Check sheet for the drawn part. Datum: minimum x, y, z corner. Units: mm. A direction names the side the tool comes from. Coordinates: 2 decimals unless noted, no trailing zeros. Loops run counter-clockwise (first coordinate to the right, second up) from the corner with the lowest first, then second, coordinate; pieces in that order, holes last.
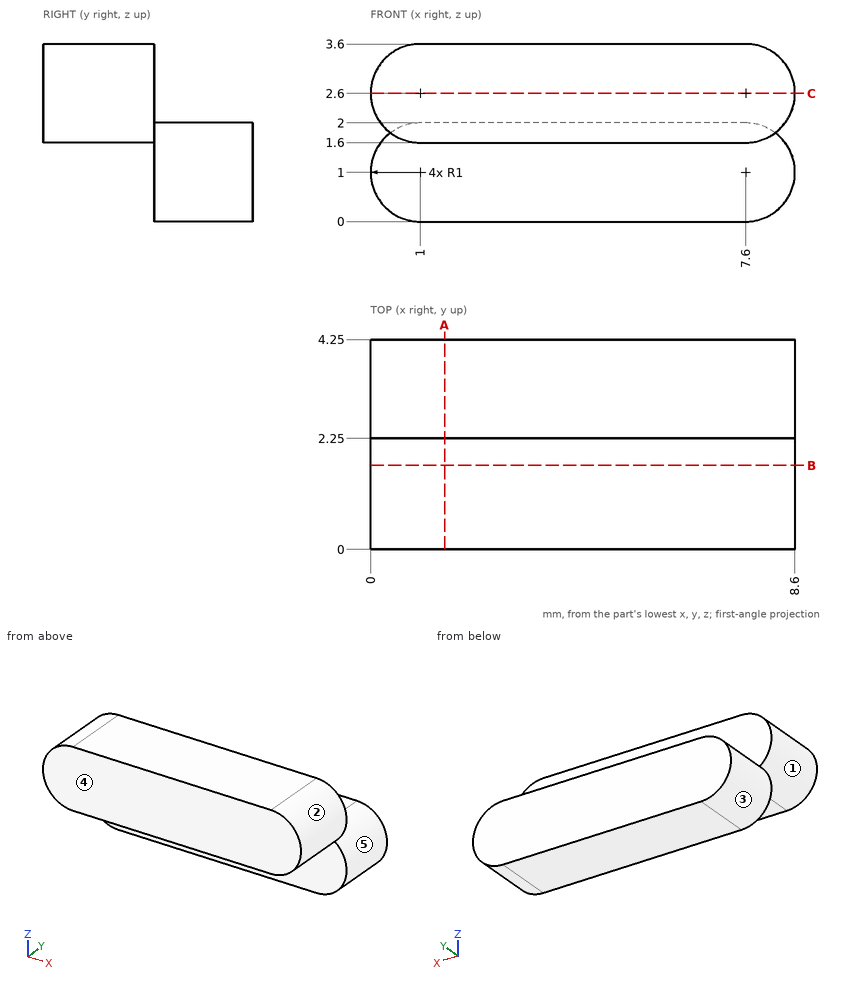
1) Section check B-B on y = 1.7. Enter the section's corners in (x, z).
Answer sheet:
outline: (1, 1.6) - (7.6, 1.6) arc R1 ccw to (7.6, 3.6) - (1, 3.6) arc R1 ccw to start
2) Section check A-A on x = 1.5. Enter the section's corners in (y, z).
Answer sheet:
outline: (0, 1.6) - (2.25, 1.6) - (2.25, 0) - (4.25, 0) - (4.25, 2) - (2.25, 2) - (2.25, 3.6) - (0, 3.6) - close
3) Depth check by flat-ended pin: pin 1 (1.1 mm diameter, centred on x = 3, y = 1, fed in from -Z); pin 2 (0.9 mm diameter, centred on x = 6, z = 3, fed in from +Y); pin 3 (1 mm diameter, centred on x = 5, y = 3, fed in from +Z); pin 4 (1 mm diameter, centred on x = 5.5, z = 3, fed in from -Y). Enter the tip coordinate at first touch or a pass-through.
Answer sheet:
pin 1: stops at z = 1.6
pin 2: stops at y = 2.25
pin 3: stops at z = 2
pin 4: stops at y = 0
4) Section check C-C on z = 2.6. Enter the section's corners in (x, y), plus the area to 4 significant figures.
Answer sheet:
outline: (0, 0) - (8.6, 0) - (8.6, 2.25) - (0, 2.25) - close
area: 19.35 mm2
5) Set-up check for the marked faces 1, 2, 3, 4 and 5: record each of +Z, -Z, +X, -X, +Y, -Y from which the full face is reachable in a straight line by a thin tool's end or side.
Answer sheet:
face 1: -X, -Y
face 2: +X, -Y
face 3: -X, +Y
face 4: +Z, -Z, +X, -X, -Y
face 5: +X, +Y
6) Scan lines: line 1 (Z direction, x = 5.5, y = 2.2); line 2 (Z direction, x = 7.5, y = 3.65); line 3 (Y direction, x = 3, z = 0.5). Record each from-to range of solid material in increasing order.
Answer sheet:
line 1: z = 1.6 to 3.6
line 2: z = 0 to 2
line 3: y = 2.25 to 4.25
